CAD build for the part. Positions are in the model's coordinates, mm. A direction names the side the tool comes from. Give positions to 0.01 mm unless a question says otherwise; leave off trailing zeros. Loops run counter-clockwise (first coordinate to the right, second up) from the corner with the lowest first, then second, coordinate; pieces in that order, holes last.
```python
from build123d import *

# Parameters (mm, degrees)
BOSS_EXTRUDE1_DEPTH           = 1
SKETCH3_W                     = 10
SKETCH3_H                     = 13.4
CUT_EXTRUDE1_DEPTH            = 98.050502317
SKETCH4_W                     = 60
SKETCH4_H                     = 1.5
BOSS_EXTRUDE3_DEPTH           = 3
SKETCH5_R                     = 2.5
BOSS_EXTRUDE4_DEPTH           = 5
BOSS_EXTRUDE4_DRAFT           = 2
BOSS_EXTRUDE4_PROFILE_2_DEPTH = 5
BOSS_EXTRUDE4_PROFILE_2_DRAFT = 2
BOSS_EXTRUDE4_PROFILE_3_DEPTH = 5
BOSS_EXTRUDE4_PROFILE_3_DRAFT = 2
BOSS_EXTRUDE4_PROFILE_4_DEPTH = 5
BOSS_EXTRUDE4_PROFILE_4_DRAFT = 2
BOSS_EXTRUDE4_PROFILE_5_DEPTH = 5
BOSS_EXTRUDE4_PROFILE_5_DRAFT = 2
BOSS_EXTRUDE4_PROFILE_6_DEPTH = 5
BOSS_EXTRUDE4_PROFILE_6_DRAFT = 2
BOSS_EXTRUDE4_PROFILE_7_DEPTH = 5
BOSS_EXTRUDE4_PROFILE_7_DRAFT = 2


with BuildPart() as part:
    # Sketch1 → Boss-Extrude1 (new body)
    with BuildSketch(Plane(origin=(0, 0, 0), x_dir=(1, 0, 0), z_dir=(0, 1, 0))):
        Polygon((63.4, 30), (86.8, 30), (86.8, 0), (63.4, 0), (63.4, -13.4), (23.4, -13.4), (23.4, 0), (0, 0), (0, 30), (23.4, 30), (23.4, 43.4), (63.4, 43.4), align=None)
    extrude(amount=BOSS_EXTRUDE1_DEPTH)

    # Sketch3 → Cut-Extrude1 (cut, through all)
    with BuildSketch(Plane(origin=(0, 1, 0), x_dir=(1, 0, 0), z_dir=(0, 1, 0))):
        Polygon((0, 0), (23.4, 0), (33.4, 0), (40.609890906, 0), (40.609890906, 5.606324955), (0, 5.606324955), align=None)
        with Locations((28.4, -6.7)):
            Rectangle(SKETCH3_W, SKETCH3_H)
        with Locations((58.4, -6.7)):
            Rectangle(SKETCH3_W, SKETCH3_H)
    extrude(amount=-CUT_EXTRUDE1_DEPTH, mode=Mode.SUBTRACT)

    # Sketch4 → Boss-Extrude3 (add)
    with BuildSketch(Plane.XZ):
        with Locations((43.4, -15.25)):
            Rectangle(SKETCH4_W, SKETCH4_H)
        with Locations((43.4, -10.75)):
            Rectangle(SKETCH4_W, SKETCH4_H)
        with Locations((43.4, -19.75)):
            Rectangle(SKETCH4_W, SKETCH4_H)
        with Locations((43.4, -24.25)):
            Rectangle(SKETCH4_W, SKETCH4_H)
    extrude(amount=BOSS_EXTRUDE3_DEPTH)


with BuildPart() as boss_extrude4_tool:
    # Sketch5 → Boss-Extrude4 (with draft: the straight prism first)
    with BuildSketch(Plane(origin=(0, 0, 0), x_dir=(-1, 0, 0), z_dir=(0, -1, 0))):
        with Locations((-4, 9.606324955)):
            Circle(SKETCH5_R)
    extrude(amount=BOSS_EXTRUDE4_DEPTH)
    # Boss-Extrude4: the draft: its side faces are tilted about the plane it starts from
    boss_extrude4_sides = [boss_extrude4_tool.faces().sort_by_distance(p)[0] for p in [
        (6.5, -2.5, -9.606324955),
    ]]
    draft(boss_extrude4_sides, Plane(origin=(0, 0, 0), x_dir=(-1, 0, 0), z_dir=(0, -1, 0)), BOSS_EXTRUDE4_DRAFT)


with BuildPart() as part_1:
    add(part.part)

    # Boss-Extrude4: add boss_extrude4_tool
    add(boss_extrude4_tool.part)


with BuildPart() as boss_extrude4_profile_2_tool:
    # Sketch5 → Boss-Extrude4 profile 2 (with draft: the straight prism first)
    with BuildSketch(Plane(origin=(0, 0, 0), x_dir=(-1, 0, 0), z_dir=(0, -1, 0))):
        with Locations((-4, 26)):
            Circle(SKETCH5_R)
    extrude(amount=BOSS_EXTRUDE4_PROFILE_2_DEPTH)
    # Boss-Extrude4 profile 2: the draft: its side faces are tilted about the plane it starts from
    boss_extrude4_profile_2_sides = [boss_extrude4_profile_2_tool.faces().sort_by_distance(p)[0] for p in [
        (6.5, -2.5, -26),
    ]]
    draft(boss_extrude4_profile_2_sides, Plane(origin=(0, 0, 0), x_dir=(-1, 0, 0), z_dir=(0, -1, 0)), BOSS_EXTRUDE4_PROFILE_2_DRAFT)


with BuildPart() as part_2:
    add(part_1.part)

    # Boss-Extrude4 profile 2: add boss_extrude4_profile_2_tool
    add(boss_extrude4_profile_2_tool.part)


with BuildPart() as boss_extrude4_profile_3_tool:
    # Sketch5 → Boss-Extrude4 profile 3 (with draft: the straight prism first)
    with BuildSketch(Plane(origin=(0, 0, 0), x_dir=(-1, 0, 0), z_dir=(0, -1, 0))):
        with Locations((-82.8, 26)):
            Circle(SKETCH5_R)
    extrude(amount=BOSS_EXTRUDE4_PROFILE_3_DEPTH)
    # Boss-Extrude4 profile 3: the draft: its side faces are tilted about the plane it starts from
    boss_extrude4_profile_3_sides = [boss_extrude4_profile_3_tool.faces().sort_by_distance(p)[0] for p in [
        (85.3, -2.5, -26),
    ]]
    draft(boss_extrude4_profile_3_sides, Plane(origin=(0, 0, 0), x_dir=(-1, 0, 0), z_dir=(0, -1, 0)), BOSS_EXTRUDE4_PROFILE_3_DRAFT)


with BuildPart() as part_3:
    add(part_2.part)

    # Boss-Extrude4 profile 3: add boss_extrude4_profile_3_tool
    add(boss_extrude4_profile_3_tool.part)


with BuildPart() as boss_extrude4_profile_4_tool:
    # Sketch5 → Boss-Extrude4 profile 4 (with draft: the straight prism first)
    with BuildSketch(Plane(origin=(0, 0, 0), x_dir=(-1, 0, 0), z_dir=(0, -1, 0))):
        with Locations((-82.8, 4)):
            Circle(SKETCH5_R)
    extrude(amount=BOSS_EXTRUDE4_PROFILE_4_DEPTH)
    # Boss-Extrude4 profile 4: the draft: its side faces are tilted about the plane it starts from
    boss_extrude4_profile_4_sides = [boss_extrude4_profile_4_tool.faces().sort_by_distance(p)[0] for p in [
        (85.3, -2.5, -4),
    ]]
    draft(boss_extrude4_profile_4_sides, Plane(origin=(0, 0, 0), x_dir=(-1, 0, 0), z_dir=(0, -1, 0)), BOSS_EXTRUDE4_PROFILE_4_DRAFT)


with BuildPart() as part_4:
    add(part_3.part)

    # Boss-Extrude4 profile 4: add boss_extrude4_profile_4_tool
    add(boss_extrude4_profile_4_tool.part)


with BuildPart() as boss_extrude4_profile_5_tool:
    # Sketch5 → Boss-Extrude4 profile 5 (with draft: the straight prism first)
    with BuildSketch(Plane(origin=(0, 0, 0), x_dir=(-1, 0, 0), z_dir=(0, -1, 0))):
        with Locations((-59.4, 39.4)):
            Circle(SKETCH5_R)
    extrude(amount=BOSS_EXTRUDE4_PROFILE_5_DEPTH)
    # Boss-Extrude4 profile 5: the draft: its side faces are tilted about the plane it starts from
    boss_extrude4_profile_5_sides = [boss_extrude4_profile_5_tool.faces().sort_by_distance(p)[0] for p in [
        (61.9, -2.5, -39.4),
    ]]
    draft(boss_extrude4_profile_5_sides, Plane(origin=(0, 0, 0), x_dir=(-1, 0, 0), z_dir=(0, -1, 0)), BOSS_EXTRUDE4_PROFILE_5_DRAFT)


with BuildPart() as part_5:
    add(part_4.part)

    # Boss-Extrude4 profile 5: add boss_extrude4_profile_5_tool
    add(boss_extrude4_profile_5_tool.part)


with BuildPart() as boss_extrude4_profile_6_tool:
    # Sketch5 → Boss-Extrude4 profile 6 (with draft: the straight prism first)
    with BuildSketch(Plane(origin=(0, 0, 0), x_dir=(-1, 0, 0), z_dir=(0, -1, 0))):
        with Locations((-27.4, 39.4)):
            Circle(SKETCH5_R)
    extrude(amount=BOSS_EXTRUDE4_PROFILE_6_DEPTH)
    # Boss-Extrude4 profile 6: the draft: its side faces are tilted about the plane it starts from
    boss_extrude4_profile_6_sides = [boss_extrude4_profile_6_tool.faces().sort_by_distance(p)[0] for p in [
        (29.9, -2.5, -39.4),
    ]]
    draft(boss_extrude4_profile_6_sides, Plane(origin=(0, 0, 0), x_dir=(-1, 0, 0), z_dir=(0, -1, 0)), BOSS_EXTRUDE4_PROFILE_6_DRAFT)


with BuildPart() as part_6:
    add(part_5.part)

    # Boss-Extrude4 profile 6: add boss_extrude4_profile_6_tool
    add(boss_extrude4_profile_6_tool.part)


with BuildPart() as boss_extrude4_profile_7_tool:
    # Sketch5 → Boss-Extrude4 profile 7 (with draft: the straight prism first)
    with BuildSketch(Plane(origin=(0, 0, 0), x_dir=(-1, 0, 0), z_dir=(0, -1, 0))):
        with Locations((-43.4, -9.4)):
            Circle(SKETCH5_R)
    extrude(amount=BOSS_EXTRUDE4_PROFILE_7_DEPTH)
    # Boss-Extrude4 profile 7: the draft: its side faces are tilted about the plane it starts from
    boss_extrude4_profile_7_sides = [boss_extrude4_profile_7_tool.faces().sort_by_distance(p)[0] for p in [
        (45.9, -2.5, 9.4),
    ]]
    draft(boss_extrude4_profile_7_sides, Plane(origin=(0, 0, 0), x_dir=(-1, 0, 0), z_dir=(0, -1, 0)), BOSS_EXTRUDE4_PROFILE_7_DRAFT)


with BuildPart() as part_7:
    add(part_6.part)

    # Boss-Extrude4 profile 7: add boss_extrude4_profile_7_tool
    add(boss_extrude4_profile_7_tool.part)


solid = part_7.part
```
1. Probe line 1 along Z through (x, y) = (63, -0.8); line 2 along X through (y, z) = (-4, -25.5); line 3 along Y through (x, z) = (46, -38.5). List the from-to ranges inside material, lowest first.
Responses:
line 1: z = -25 to -23.5, -20.5 to -19, -16 to -14.5, -11.5 to -10
line 2: x = 1.69 to 6.31, 80.49 to 85.11
line 3: y = 0 to 1
2. Saw through at B-B, the plane z = 9.4. List the corners of the cut face in (x, y), and give its area (3 significant figures).
Responses:
outline: (33.4, 0) - (40.9, 0) - (41.07, -5) - (45.73, -5) - (45.9, 0) - (53.4, 0) - (53.4, 1) - (33.4, 1) - close
area: 44.1 mm2
3. Saw through at C-C, the plane x = 71. List the corners of the cut face in (y, z), and give its area (3 significant figures).
Responses:
outline: (-3, -25) - (0, -25) - (0, -30) - (1, -30) - (1, 0) - (0, 0) - (0, -10) - (-3, -10) - (-3, -11.5) - (0, -11.5) - (0, -14.5) - (-3, -14.5) - (-3, -16) - (0, -16) - (0, -19) - (-3, -19) - (-3, -20.5) - (0, -20.5) - (0, -23.5) - (-3, -23.5) - close
area: 48.0 mm2
4. Pull direction Z, two halves, no side cores. Call faces 1 (the face through (4, -5, -26)), 2 (the face through (44, 0, -22)): released by +Z, released by -Z, zero draft, split by the parting line, or undercut.
Responses:
face 1: zero draft
face 2: undercut
5. Saw through at A-A, the plane x = 43.4. List the corners of the cut face in (y, z), and give its area (3 significant figures).
Responses:
outline: (-5, 7.07) - (0, 6.9) - (0, -10) - (-3, -10) - (-3, -11.5) - (0, -11.5) - (0, -14.5) - (-3, -14.5) - (-3, -16) - (0, -16) - (0, -19) - (-3, -19) - (-3, -20.5) - (0, -20.5) - (0, -23.5) - (-3, -23.5) - (-3, -25) - (0, -25) - (0, -43.4) - (1, -43.4) - (1, 13.4) - (0, 13.4) - (0, 11.9) - (-5, 11.73) - close
area: 98.9 mm2
6. Drop flat-ended pins along their axis: pin 1 (0.5 mm diameter, centred on y = 0.5, z = 9, fed in from -X); pin 2 (2.5 mm diameter, centred on x = 55, y = -1.5, fed in from -Z); pin 3 (1.6 mm diameter, centred on y = -1, z = -15, fed in from +X). Give the stop position or say it passes through.
Responses:
pin 1: stops at x = 33.4
pin 2: stops at z = -25
pin 3: stops at x = 73.4
7. Saw through at D-D, the plane z = -4. List the corners of the cut face in (x, y), and give its area (3 significant figures).
Responses:
outline: (40.61, 0) - (80.3, 0) - (80.47, -5) - (85.13, -5) - (85.3, 0) - (86.8, 0) - (86.8, 1) - (40.61, 1) - close
area: 70.3 mm2
8. Tool access for faces 3 (the face through (84.716, -2.465, -2.531)), 4 (the face through (43, -1, -14.5)), 5 (the face through (27, -5, -39)), 6 (the face through (43, -1, -11.5)): list every direction of +Z, -Z, +X, -X, +Y, -Y with a clear straight run to the whole face (end or side of a thin tool).
Responses:
face 3: -Y
face 4: +X, -X, -Y
face 5: +Z, -Z, +X, -X, -Y
face 6: +X, -Y
